from build123d import *

# Parameters (mm, degrees)
F1_DEPTH = 10


with BuildPart() as f1:
    # F0 (on Top) → F1 (new body)
    with BuildSketch(Plane.XY):
        Polygon((-55.302736, 7.375862), (-58.234972, 6.376695), (-60.152077, 5.339073), (-60.879436, 4.272422), (-60.465326, 3.256186), (-59.146603, 2.608351), (-57.060198, 2.280282), (-51.132099, 2.388886), (-47.564265, 2.728284), (-43.776487, 3.192897), (-39.9057, 3.734085), (-36.088835, 4.303211), (-32.462829, 4.851638), (-29.16461, 5.330727), (-26.331116, 5.691841), (-24.190234, 5.753123), (-22.194411, 5.477108), (-20.343403, 4.916947), (-18.636961, 4.125795), (-17.074837, 3.156806), (-15.656783, 2.063133), (-14.382549, 0.897931), (-13.251887, -0.285646), (-12.26455, -1.434445), (-11.420288, -2.495312), (-10.718854, -3.415091), (-10.159999, -4.140631), (-9.524376, -4.828129), (-8.788524, -5.439376), (-7.97831, -5.964872), (-7.119602, -6.395116), (-6.238268, -6.720607), (-5.360175, -6.931844), (-4.511192, -7.019325), (-3.717186, -6.97355), (-3.004025, -6.785017), (-2.397576, -6.444227), (-1.923709, -5.941677), (-1.60829, -5.267867), (-1.316886, -4.342745), (-1.022677, -3.48605), (-0.73894, -2.704866), (-0.478953, -2.006273), (-0.255994, -1.397351), (-0.083341, -0.885182), (0.025728, -0.476847), (0.057934, -0.179426), (0, 0), (-0.439399, -0.023458), (-0.847422, -0.240503), (-1.750059, -0.642884), (-2.380218, -0.628156), (-2.764398, -0.266297), (-2.929102, 0.372723), (-2.900829, 1.21893), (-2.706082, 2.202353), (-2.371363, 3.253021), (-1.923173, 4.300961), (-1.388014, 5.276201), (-0.792387, 6.108769), (-0.162794, 6.728694), (0.474264, 7.066004), (1.556662, 7.323265), (2.680252, 7.520912), (3.8367, 7.665848), (5.017661, 7.764977), (6.214798, 7.825203), (7.41977, 7.853431), (8.624236, 7.856563), (9.819855, 7.841504), (10.998289, 7.815158), (12.151196, 7.784429), (13.270234, 7.75622), (14.347066, 7.737436), (15.250982, 7.729441), (15.954305, 7.727012), (16.512773, 7.72817), (16.982119, 7.730942), (17.876389, 7.733422), (18.412779, 7.72918), (19.082985, 7.718649), (19.942745, 7.699855), (21.047785, 7.670821), (22.453844, 7.629573), (24.216658, 7.574135), (24.588085, 7.498381), (24.926546, 7.307823), (25.234154, 7.019938), (25.513015, 6.652199), (25.765228, 6.222079), (25.992907, 5.747053), (26.198155, 5.244594), (26.383079, 4.732176), (26.549778, 4.227272), (26.700369, 3.747357), (26.836949, 3.309903), (26.961631, 2.932385), (27.13333, 2.579536), (27.369267, 2.30779), (27.656524, 2.13622), (27.982178, 2.083901), (28.333305, 2.169907), (28.696983, 2.413315), (29.060288, 2.833197), (29.410294, 3.44863), (29.734078, 4.278687), (30.01872, 5.342444), (30.251293, 6.658976), (30.418883, 8.247355), (30.016276, 10.015402), (28.598833, 11.396484), (26.299964, 12.432229), (23.253067, 13.164268), (19.591554, 13.634228), (15.448823, 13.883739), (10.958283, 13.954428), (6.253337, 13.887925), (1.467391, 13.725859), (-3.266151, 13.509857), (-7.813885, 13.281547), (-12.042406, 13.08256), (-16.253359, 12.853671), (-21.020672, 12.501489), (-26.169738, 12.035443), (-31.525944, 11.464957), (-36.914683, 10.799458), (-42.161341, 10.048373), (-47.09131, 9.221129), (-51.529978, 8.327149), align=None)
    extrude(amount=F1_DEPTH)


solid = f1.part
Work out the finished part from the listing and answer in its coordinate system (mm). A direction names the side the tool comes from. Round coordinates to 2 decimals unless told otherwise and drop trailing zeros. Answer as CSV lines item,"result". Start each with the question number.
(1) Find the intervals of material crossed by probe 1 along Y at (x, z) = (1.5, 4.5); probe 2 along Y at (x, z) = (20.5, 8.5); probe 3 along X at (y, z) = (-3.5, 7.75), in increasing order.
(2) Each of these flat-tipped pins is pushed along its axis until it touches: pin 1 (8 mm diameter, centred on x = -24, y = -2, fed in from +Z); pin 2 (4 mm diameter, centred on y = 2.5, z = 6, fed in from +X); pin 3 (1.5 mm diameter, centred on x = -29, z = 2.5, fed in from -Y). Where does it stop, or does it pass through?
(3) The mould has two halves that part along X. Classify faces 3 (the flat face through (-38.024, 4.015, 4.93)), 4 (the flat face through (-39.5, 10.43, 4.93)), 5 (the flat face through (-16, 6, 0)), 6 (the flat face through (27.465, 11.907, 4.93)): +X half, -X half, draft (parallel to the pull), parting line (faces both ways), or undercut.
(4) A tool of negligible diameter and unlimited length cuts with its end or side. For faces 1 (the flat face through (-45.697, 2.957, 4.93)), 2 (the flat face through (-44.59, 9.64, 4.93)), from which of +Z, -Z, +X, -X, +Y, -Y can it reach the whole face along a straight path? Write none if from no direction.
Output values:
1,probe 1,"y = 7.31 to 13.73"
1,probe 2,"y = 7.69 to 13.52"
1,probe 3,"x = -10.65 to -1.03"
2,pin 1,"passes through"
2,pin 2,"stops at x = 29.79"
2,pin 3,"stops at y = 5.25"
3,face 3,"undercut"
3,face 4,"-X half"
3,face 5,"draft"
3,face 6,"+X half"
4,face 1,"+Z, -Z, -Y"
4,face 2,"+Z, -Z, -X, +Y"
